from build123d import *


with BuildPart() as f1:
    # F0 (on Front) → F1 (revolve)
    with BuildSketch(Plane.XZ):
        with BuildLine():
            Line((0, 23.8125), (0, 0))
            Line((0, 0), (18.826609, 0))
            ThreePointArc((18.826609, 0), (19.668508, 0.348726), (20.017234, 1.190625))
            Line((20.017234, 1.190625), (20.017234, 2.38125))
            Line((20.017234, 2.38125), (15.009553, 2.38125))
            ThreePointArc((15.009553, 2.38125), (9.744412, 4.147372), (6.609293, 8.73125))
            Line((6.609293, 8.73125), (5.159375, 8.73125))
            ThreePointArc((5.159375, 8.73125), (6.35, 9.921875), (5.159375, 11.1125))
            Line((5.159375, 11.1125), (3.175, 11.1125))
            Line((3.175, 11.1125), (3.175, 23.8125))
            Line((3.175, 23.8125), (0, 23.8125))
        make_face()
    revolve(axis=Axis((0, 0, 11.90625), (0, 0, 1)))


solid = f1.part
Model file for the job. Use its own axes, mm. A direction names the side the tool comes from. Give positions to 0.01 mm unless a question says otherwise; leave off trailing zeros. Loops run counter-clockwise (first coordinate to the right, second up) from the corner with the lowest first, then second, coordinate; pieces in that order, holes last.
Item 1: Slice it at C-C (z = 12). Write the cut outline in (x, y) (3 decimals), plus the area to 3 significant figures.
Check values:
outline: circle Ø6.35 at (0, 0)
area: 31.7 mm2
Item 2: Which spindle directions (+Z, -Z, +X, -X, +Y, -Y) get a long thin tool onto all of the face, cutting with end or side? Do faces 1 (the face through (-0.69, -3.1, 17.55)), 2 (the face through (0, 0, 0)). Say none if no direction does.
Check values:
face 1: +Z
face 2: -Z, +X, -X, +Y, -Y
Item 3: Drill centre lines: line 1 along Z through (x, y) = (7.5, -15.5); line 2 along X through (y, z) = (-1.5, 6); line 3 along Z through (x, y) = (3.5, -7.5). Where is each one in solid material? Low to high.
Check values:
line 1: z = 0 to 2.38
line 2: x = -7.79 to 7.79
line 3: z = 0 to 5.55
Item 4: Drop flat-ended pins along their axis: P1, Ø8, axis at y = -2, z = 14, coming from the +X side; P2, Ø3, axis at y = 1, z = 13.5, coming from the +X side (3 decimals); P3, Ø3, axis at x = 15.5, y = 9.5, coming from the -Z side; P4, Ø8, axis at x = 16, y = 6, coming from the +Z side. Give the stop position or say it passes through.
Check values:
P1: stops at x = 6.27
P2: stops at x = 3.175
P3: stops at z = 0
P4: stops at z = 2.6
Item 5: Slice it at D-D (z = 4.25). Write the cut outline in (x, y).
Check values:
outline: circle Ø19.22 at (0, 0)
Item 6: Slice it at A-A (y = 0). Write the cut outline in (x, z) (1 decimal), plus the area to 3 significant figures.
Check values:
outline: (-20, 1.2) arc R1.2 ccw to (-18.8, 0) - (18.8, 0) arc R1.2 ccw to (20, 1.2) - (20, 2.4) - (15, 2.4) arc R8.7 cw to (6.6, 8.7) - (5.2, 8.7) arc R1.2 ccw to (5.2, 11.1) - (3.2, 11.1) - (3.2, 23.8) - (-3.2, 23.8) - (-3.2, 11.1) - (-5.2, 11.1) arc R1.2 ccw to (-5.2, 8.7) - (-6.6, 8.7) arc R8.7 cw to (-15, 2.4) - (-20, 2.4) - close
area: 316 mm2
